from build123d import *

# Parameters (mm, degrees)
F0_R     = 19.65
F1_DEPTH = 6
F2_R     = 16.1
F3_DEPTH = 25
F4_SIZE2 = 2
F4_SIZE  = 0.8
F5_SIZE2 = 2
F5_SIZE  = 0.8


with BuildPart() as f1:
    # F0 (on Top) → F1 (new body)
    with BuildSketch(Plane.XY):
        Circle(F0_R)
    extrude(amount=F1_DEPTH)

    # F2 (on face) → F3 (cut)
    with BuildSketch(Plane.XY.offset(6)):
        Circle(F2_R)
    extrude(amount=-F3_DEPTH, mode=Mode.SUBTRACT)

    # F4
    f4_edges = [f1.edges().sort_by_distance(p)[0] for p in [
        (-16.1, 0, 0),
    ]]
    chamfer(f4_edges, length=F4_SIZE, length2=F4_SIZE2)

    # F5
    f5_edges = [f1.edges().sort_by_distance(p)[0] for p in [
        (-19.65, 0, 6),
    ]]
    f5_side = f1.faces().sort_by_distance((-19.094214, 0, 6))[0]
    chamfer(f5_edges, length=F5_SIZE, length2=F5_SIZE2, reference=f5_side)


solid = f1.part
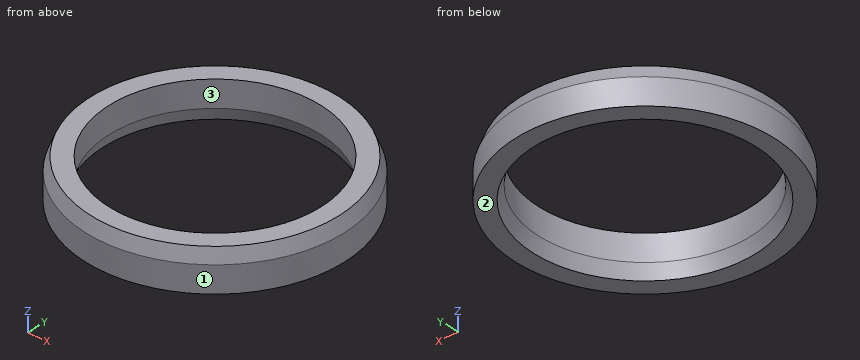
Read the model definition and answer for the solid it produces. Units are mm, in the model's axes. Face numbers are marked on the shaded views. Round coordinates to 2 decimals unless told otherwise and drop trailing zeros. Write each loop counter-clockwise with the first axis right and the second up, starting at its lowest first coordinate (ties: lowest second). Pieces come first, ordered by that corner, then holes.
Q1. Find section A-A on x = 0. Determine the outline of the cut face in (y, z).
Values:
outline: (-19.65, 0) - (-16.9, 0) - (-16.1, 2) - (-16.1, 6) - (-18.85, 6) - (-19.65, 4) - close; (16.1, 2) - (16.9, 0) - (19.65, 0) - (19.65, 4) - (18.85, 6) - (16.1, 6) - close
Q2. The mould has two halves that part along Y. Classify the marked faces 1, 2 and 3: released by +Y, released by -Y, zero draft, split by the parting line, or undercut.
Values:
face 1: split by the parting line
face 2: zero draft
face 3: undercut
Q3. Find section C-C on z = 0.9. Determine the outline of the cut face in (x, y).
Values:
outline: circle Ø39.3 at (0, 0); hole circle Ø33.08 at (0, 0)
Q4. Straight lines are drawn through the part: line 1 (Y direction, x = 0, z = 3.7); line 2 (X direction, y = 2.5, z = 1.5); line 3 (Y direction, x = -4, z = 5.3). For each, find the intervals that lie inside material, in ascending order.
Values:
line 1: y = -19.65 to -16.1, 16.1 to 19.65
line 2: x = -19.49 to -16.11, 16.11 to 19.49
line 3: y = -18.71 to -15.6, 15.6 to 18.71
Q5. Flat-ended cylindrical pins translate along their axes: P1, Ø2, axis at x = -0.5, z = 1, coming from the -Y side; P2, Ø1.5, axis at y = 11.5, z = 4, coming from the -X side. Find the tip coordinate at first contact, or state that the pin passes through.
Values:
P1: stops at y = -19.65
P2: stops at x = -16.45
Q6. Find section D-D on z = 5.3. Determine the outline of the cut face in (x, y).
Values:
outline: circle Ø38.26 at (0, 0); hole circle Ø32.2 at (0, 0)
